The figure shows three views and two pictorial views of one solid part (mm, origin at its lowest corner). Answer the questions. A direction names the side the tool comes from. Give positions to 0.01 mm unless a question says otherwise; leave off trailing zeros. Loops run counter-clockwise (first coordinate to the right, second up) from the corner with the lowest first, then second, coordinate; pieces in that order, holes last. Notation, with made-up numbers: (-17, -17.75) - (15, -17.75) arc R31 cw to (15, 11.25) - close; hole circle Ø7 at (16, 35). An arc over 180 degrees is marked (long way). Write each question's results on one line, items separated by ' | '.
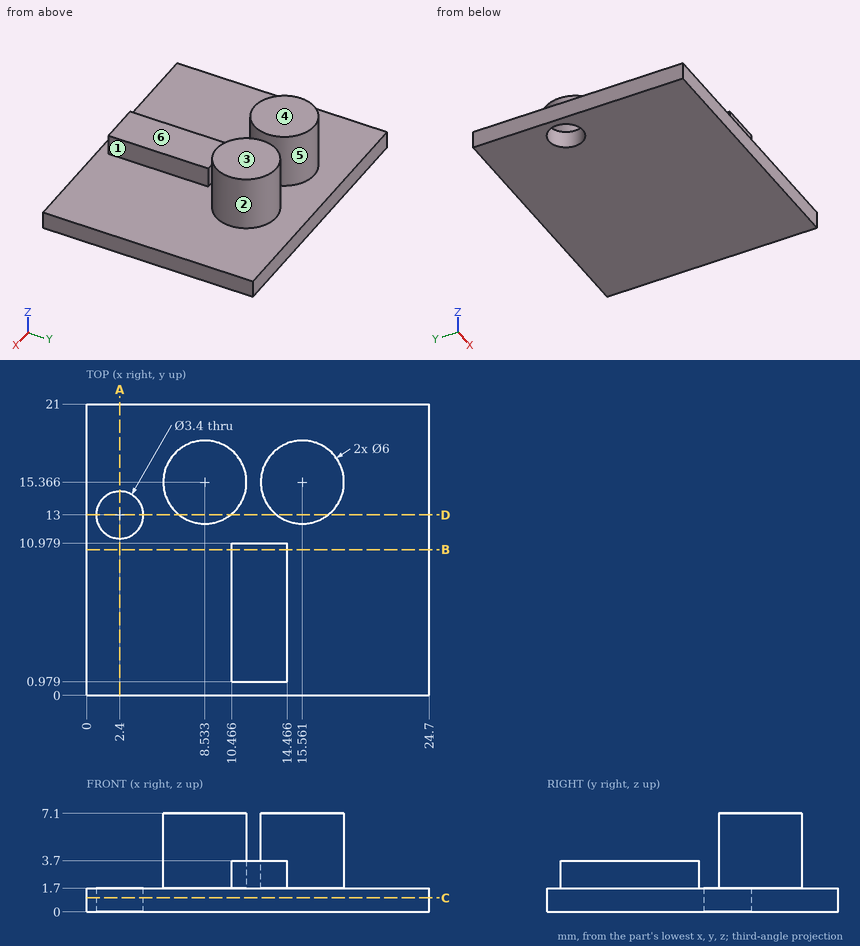
Item 1: A cutting plane is placed at B-B, the plane y = 10.5. Determine the outline of the cut face in (x, z) (1 decimal).
Values found:
outline: (0, 0) - (24.7, 0) - (24.7, 1.7) - (14.5, 1.7) - (14.5, 3.7) - (10.5, 3.7) - (10.5, 1.7) - (0, 1.7) - close
Item 2: A cutting plane is placed at A-A, the plane x = 2.4. Determine the outline of the cut face in (y, z).
Values found:
outline: (0, 0) - (11.3, 0) - (11.3, 1.7) - (0, 1.7) - close; (14.7, 0) - (21, 0) - (21, 1.7) - (14.7, 1.7) - close
Item 3: For the marked faces 4, 5 and 6, determine the directions among +Z, -Z, +X, -X, +Y, -Y from which every point of the face is accessible in a straight line to the end or side of a thin tool.
Values found:
face 4: +Z, +X, -X, +Y, -Y | face 5: +Z | face 6: +Z, +X, -X, -Y
Item 4: A cutting plane is placed at D-D, the plane y = 13. Determine the outline of the cut face in (x, z) (1 decimal).
Values found:
outline: (0, 0) - (0.7, 0) - (0.7, 1.7) - (0, 1.7) - close; (4.1, 0) - (24.7, 0) - (24.7, 1.7) - (17.4, 1.7) - (17.4, 7.1) - (13.7, 7.1) - (13.7, 1.7) - (10.4, 1.7) - (10.4, 7.1) - (6.7, 7.1) - (6.7, 1.7) - (4.1, 1.7) - close
Item 5: Flat-ended cylindrical pins translate along their axes: P1, Ø0.6, axis at y = 7, z = 3, coming from the -X side; P2, Ø8, axis at x = 16.5, y = 4.5, coming from the +Z side; P3, Ø1.5, axis at y = 13.5, z = 5.5, coming from the +X side (1 decimal). Find the tip coordinate at first contact, or state that the pin passes through.
Values found:
P1: stops at x = 10.47 | P2: stops at z = 3.7 | P3: stops at x = 18.3
Item 6: For a pull along X with two mould halves and no side action, classify the marked faces 1, 2 and 3 as released by +X, released by -X, zero draft, split by the parting line, or undercut.
Values found:
face 1: released by +X | face 2: undercut | face 3: zero draft
Item 7: A cutting plane is placed at C-C, the plane z = 1. Determine the outline of the cut face in (x, y).
Values found:
outline: (0, 0) - (24.7, 0) - (24.7, 21) - (0, 21) - close; hole circle Ø3.4 at (2.4, 13)
Item 8: Find the intervals of material crossed by line 1 along X through (y, z) = (13, 1.2); line 2 along Y through (x, z) = (2.4, 0.95); line 3 along Z through (x, y) = (7.5, 19.75), in increasing order. Write a range as [from, to].
Values found:
line 1: x = [0, 0.7], [4.1, 24.7] | line 2: y = [0, 11.3], [14.7, 21] | line 3: z = [0, 1.7]
